```python
from build123d import *

# Parameters (mm, degrees)
SKETCH1_W           = 51.3
SKETCH1_H           = 43.5
BOSS_EXTRUDE1_DEPTH = 3
SKETCH2_W           = 12
SKETCH2_H           = 12
CUT_EXTRUDE1_DEPTH  = 3
SKETCH3_W           = 10
SKETCH3_H           = 43.5
BOSS_EXTRUDE2_DEPTH = 1.7
CHAMFER1_SIZE       = 1
SKETCH4_R           = 0.6


with BuildPart() as part:
    # Sketch1 → Boss-Extrude1 (new body)
    with BuildSketch(Plane(origin=(0, 0, 0), x_dir=(1, 0, 0), z_dir=(0, 1, 0))):
        Rectangle(SKETCH1_W, SKETCH1_H)
    extrude(amount=BOSS_EXTRUDE1_DEPTH)

    # Sketch2 → Cut-Extrude1 (cut)
    with BuildSketch(Plane(origin=(0, 3, 0), x_dir=(1, 0, 0), z_dir=(0, 1, 0))):
        with Locations((-5.65, 0.05)):
            Rectangle(SKETCH2_W, SKETCH2_H)
    extrude(amount=-CUT_EXTRUDE1_DEPTH, mode=Mode.SUBTRACT)

    # Sketch3 → Boss-Extrude2 (add)
    with BuildSketch(Plane(origin=(0, 3, 0), x_dir=(1, 0, 0), z_dir=(0, 1, 0))):
        with Locations((20.65, 0)):
            Rectangle(SKETCH3_W, SKETCH3_H)
    extrude(amount=BOSS_EXTRUDE2_DEPTH)

    # Chamfer1
    chamfer1_edges = [part.edges().sort_by_distance(p)[0] for p in [
        (15.65, 4.7, 0),
    ]]
    chamfer(chamfer1_edges, length=CHAMFER1_SIZE)

    # handle: sweep along a path in Sketch5
    with BuildLine(Plane(origin=(0, 3, 0), x_dir=(1, 0, 0), z_dir=(0, 1, 0))) as handle_path:
        Line((20.68654036, -21.75), (20.68654036, -22.031235757))
        ThreePointArc((20.68654036, -22.031235757), (20.393647141, -22.738342538), (19.68654036, -23.031235757))
        Line((19.68654036, -23.031235757), (-28.502744804, -23.031235757))
    # Sketch4 → handle (sweep)
    with BuildSketch(Plane.XY.offset(21.75)):
        with Locations((20.68654036, 2.094896924)):
            Circle(SKETCH4_R)
    sweep(path=handle_path.line)


solid = part.part
```
CAD build for the part. Positions are in the model's coordinates, mm. A direction names the side the tool comes from. Round coordinates to 2 decimals unless told otherwise and drop trailing zeros. Order: outer loops, then holes, each group sorted by start corner. A loop starts at its lowest first (then second) coordinate and runs counter-clockwise, first axis right, second up. Notation, with made-up numbers: (86.5, 37) - (94.5, 37) arc R20 ccw to (94.5, 49) - close; hole circle Ø6 at (-37.5, 3). An arc over 180 degrees is marked (long way). Answer as CSV lines item,"result". Start each with the question number.
1. Pin check, flat tips, straight feed: pin 1 (1 mm diameter, centred on x = 8.5, z = -7, fed in from +Y); pin 2 (2.5 mm diameter, centred on y = 1.5, z = -1, fed in from -X). Stop position of each tip, or through.
2. Saw through at B-B, the plane x = -10. Write the cut outline in (y, z).
3. Drill centre lines: L1, parallel to Z at x = -7, y = 2.05; L2, parallel to Z at x = 22.5, y = 3.3; L3, parallel to X at y = 1, z = 5. Where is each one in solid material? Low to high. Write a range as [from, to].
4. Saw through at A-A, the plane z = 1. Write the cut outline in (x, y).
5. Saw through at C-C, the plane z = 17. Write the cut outline in (x, y).
6. Saw through at D-D, the plane x = -23.5. Write the cut outline in (y, z), and give its area (3 significant figures).
7. Pull direction Z, two halves, no side cores. Call faces 1 (the face through (0, 2, -21.75)), 2 (the face through (-6, 2, -6.05)), 3 (the face through (21, 4.7, 0)): +Z half, -Z half, draft (parallel to the pull), parting line (faces both ways), or undercut.
8. Tool access for faces 4 (the face through (-25.65, 1, 0)), 5 (the face through (-6, 2, 5.95)), 6 (the face through (-14, 3, 0)), 7 (the face through (-4.7, 1.9, 23.6)): list every direction of +Z, -Z, +X, -X, +Y, -Y with a clear straight run to the whole face (end or side of a thin tool).
Model answer:
1,pin 1,"stops at y = 3"
1,pin 2,"stops at x = -25.65"
2,outline,"(0, -21.75) - (3, -21.75) - (3, -6.05) - (0, -6.05) - close; (0, 5.95) - (3, 5.95) - (3, 21.75) - (0, 21.75) - close; circle Ø1.2 at (2.09, 23.03)"
3,L1,"z = [-21.75, -6.05], [5.95, 21.75], [22.43, 23.63]"
3,L2,"z = [-21.75, 21.75]"
3,L3,"x = [-25.65, -11.65], [0.35, 25.65]"
4,outline,"(-25.65, 0) - (-11.65, 0) - (-11.65, 3) - (-25.65, 3) - close; (0.35, 0) - (25.65, 0) - (25.65, 4.7) - (16.65, 4.7) - (15.65, 3.7) - (15.65, 3) - (0.35, 3) - close"
5,outline,"(-25.65, 0) - (25.65, 0) - (25.65, 4.7) - (16.65, 4.7) - (15.65, 3.7) - (15.65, 3) - (-25.65, 3) - close"
6,outline,"(0, -21.75) - (3, -21.75) - (3, 21.75) - (0, 21.75) - close; circle Ø1.2 at (2.09, 23.03)"
6,area,"132 mm²"
7,face 1,"-Z half"
7,face 2,"undercut"
7,face 3,"draft"
8,face 4,"-Z, -X, +Y, -Y"
8,face 5,"+Y, -Y"
8,face 6,"+Z, -Z, -X, +Y"
8,face 7,"-X"
